Source: CAD feature listing. Evaluate the final solid. Frame: model axes, mm. Face numbers are marked on the shaded views. Give positions to 0.01 mm unless a question says otherwise; leave off trailing zeros. Loops run counter-clockwise (first coordinate to the right, second up) from the corner with the lowest first, then second, coordinate; pieces in that order, holes last. Notation, with made-up numbers: M 39.5,62 L 82.5,62 A10 cw 82.5,66 Z; hole C 43,46 d3. An arc over 180 degrees is marked long. Answer in a Markdown table with one row per item.
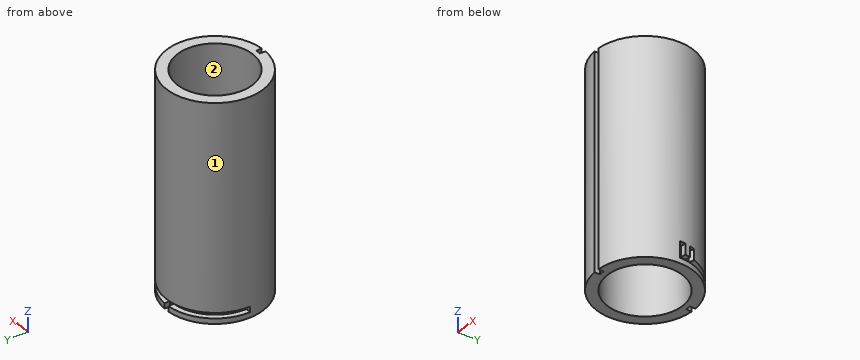
Autodesk Inventor part; units mm, degrees
ref_plane "YZ Plane" through (0, 0, 0) normal (1, 0, 0) x (0, 1, 0)
ref_plane "XZ Plane" through (0, 0, 0) normal (0, 1, 0) x (-1, 0, 0)
ref_plane "XY Plane" through (0, 0, 0) normal (0, 0, 1) x (1, 0, 0)
sketch "Sketch1" plane through (0, 0, 0) normal (0, 0, 1) x (1, 0, 0)
  circle A0 centre (0, 0) radius 25.4
  circle A1 centre (0, 0) radius 22.225
  line L0 (0, 0) -> (0, 25.4)
  line L1 (0, 0) -> (19.2474, -11.1125)
  line L2 (0, 0) -> (-19.2474, -11.1125)
  line L3 (-19.2474, -11.1125) -> (-21.997, -12.7)
  line L4 (19.2474, -11.1125) -> (21.997, -12.7)
  arc A2 (9.6237, 23.5063) -> (-9.6237, 23.5063) centre (0, 0) ccw
  arc A3 (2.54, 25.2727) -> (-2.54, 25.2727) centre (0, 0) ccw
  arc A4 (21.2995, -13.8381) -> (22.9699, -10.8419) centre (0, 0) ccw
  arc A5 (20.5909, -14.872) -> (23.1385, -10.477) centre (0, 0) ccw
  dimension "d0" = 50.8
  dimension "d1" = 44.45
  dimension "d2" = 120
  dimension "d3" = 120
  dimension "d5" = 25.4
extrude "Extrusion1" add sketch "Sketch1" along normal blind 127 contours A0 L4 A1 L0 | L0 A1 L3 A0 | A0 L3 A1 L4
sketch "Sketch9" plane through (0, 0, 127) normal (0, 0, 1) x (1, 0, 0)
  circle A0 centre (0, 0) radius 28.575
  circle A1 centre (0, 0) radius 25.4
  circle A2 centre (0, 0) radius 25.4
  arc A3 (1.4111, 25.3608) -> (-1.4111, 25.3608) centre (0, 0) ccw
  line L0 (1.5875, 28.5309) -> (1.4111, 25.3608)
  line L1 (-1.4111, -25.3608) -> (-1.5875, -28.5309)
  line L2 (-1.5875, 28.5309) -> (-1.4111, 25.3608)
  line L3 (1.4111, -25.3608) -> (1.5875, -28.5309)
  point P0 (-1.4111, 25.3608)
  dimension "d62" = 57.15
extrude "Extrusion7" add sketch "Sketch9" against normal blind 127 contours A0 L3 A1 L0 | L2 A1 L1 A0
extrude "Extrusion8" add sketch "Sketch9" against normal blind 120.65 contours L0 A1 L2 A0
ref_plane "Work Plane7" through (0, 0, 6.35) normal (0, 0, -1) x (-1, 0, 0)
sketch "Sketch10" plane through (0, 0, 6.35) normal (0, 0, -1) x (-1, 0, 0)
  circle A0 centre (0, 0) radius 25.4
  circle A1 centre (0, 0) radius 28.575
  line L0 (1.4111, -25.3608) -> (1.5875, -28.5309)
  line L1 (0, 0) -> (28.575, 0)
  arc A2 (1.5875, -28.5309) -> (1.5875, 28.5309) centre (0, 0) ccw
  line L2 (0, 0) -> (-28.575, 0)
  arc A3 (1.5875, -28.5309) -> (-1.5875, -28.5309) centre (0, 0) ccw
  line L3 (1.5875, 28.5309) -> (0, 0)
  line L4 (0, 0) -> (-1.5875, 28.5309)
  point P0 (25.4, 0)
  point P1 (-25.4, 0)
  point P2 (1.4111, 25.3608)
  point P3 (-1.4111, 25.3608)
extrude "Extrusion10" cut sketch "Sketch10" along normal blind 3.175 contours A0 L3 A1 L1 | L2 A1 L4 A0
sketch "Sketch11" plane through (0, 0, 6.35) normal (0, 0, -1) x (-1, 0, 0)
  line L0 (-28.575, 0) -> (-25.4, 0)
  line L1 (0, 0) -> (-28.575, 0)
  line L2 (-28.575, 0) -> (0, 0)
  arc A0 (28.575, 0) -> (-28.575, 0) centre (0, 0) ccw
  line L3 (-28.575, 0) -> (-28.3986, 3.1701)
  arc A1 (-1.5875, 28.5309) -> (-1.5875, -28.5309) centre (0, 0) ccw
  line L4 (-28.3986, 3.1701) -> (0, 0)
  line L5 (-28.3986, 3.1701) -> (-27.8716, 6.3011)
  line L6 (-27.8716, 6.3011) -> (-27.0005, 9.3542)
  line L7 (0, 0) -> (-27.8716, 6.3011)
  line L8 (-27.0005, 9.3542) -> (0, 0)
  arc A2 (-1.4111, -25.3608) -> (1.4111, -25.3608) centre (0, 0) ccw
  circle A3 centre (0, 0) radius 25.4
  point P0 (-24.7748, 5.6009)
  point P1 (-24.0005, 8.3149)
  point P2 (-25.2432, 2.8179)
  dimension "d77" = 3.175
  dimension "d78" = 3.175
  dimension "d79" = 3.175
extrude "Extrusion11" cut sketch "Sketch11" against normal blind 6.35 contours L3 L4 A3 L0 | A0 L3 | A0 L6 | L6 L8 A3 L7
properties part number "Maze"
Q1. Section query A-A (x = 0). Output: boundary loops of the cut face in (y, z) (3 decimals), plus the area to 3 significant figures.
Values follow:
| item | result |
|---|---|
| outline | M -25.4,0 L -22.225,0 L -22.225,127 L -25.4,127 Z; M 22.225,0 L 25.4,0 L 25.4,6.35 L 28.575,6.35 L 28.575,127 L 22.225,127 Z |
| area | 1,190 mm^2 |
Q2. Section query C-C (x = -8). Output: boundary loops of the cut face in (y, z) (3 decimals), plus the area to 3 significant figures.
Values follow:
| item | result |
|---|---|
| outline | M -27.432,0 L -20.735,0 L -20.735,127 L -27.432,127 Z; M 20.735,0 L 27.432,0 L 27.432,3.175 L 24.107,3.175 L 24.107,6.35 L 27.432,6.35 L 27.432,127 L 20.735,127 Z |
| area | 1,690 mm^2 |
Q3. Contact query for flat-ended pins moving along their axis: pin 1 Ø3 at (y, z) = (-15.5, 46.5) entering from +X; pin 2 Ø1.5 at (x, z) = (8, 94.5) entering from +Y; pin 3 Ø1.5 at (x, z) = (14.5, 72) entering from +Y. Output: stop coordinate, or through.
Values follow:
| item | result |
|---|---|
| pin 1 | x = 24.91 |
| pin 2 | y = 27.64 |
| pin 3 | y = 25.05 |
Q4. Mould query, pull axis X, two halves, no side actions, for the marked faces 1 and 2. Classes: +X half, -X half, draft (parallel to the pull), parting line (faces both ways), or undercut.
Values follow:
| item | result |
|---|---|
| face 1 | parting line |
| face 2 | undercut |
Q5. Ray query, probe 1 along X at (y, z) = (0, 27) (3 decimals); probe 2 along Z at (x, y) = (12, 23) (3 decimals); probe 3 along Y at (x, z) = (0, 48) (3 decimals). Return the intervals inside material, ascending. Write a range as from..to.
Values follow:
| item | result |
|---|---|
| probe 1 | -28.575..-22.225, 22.225..28.575 |
| probe 2 | 0..3.175, 6.35..127 |
| probe 3 | -25.4..-22.225, 22.225..28.575 |
